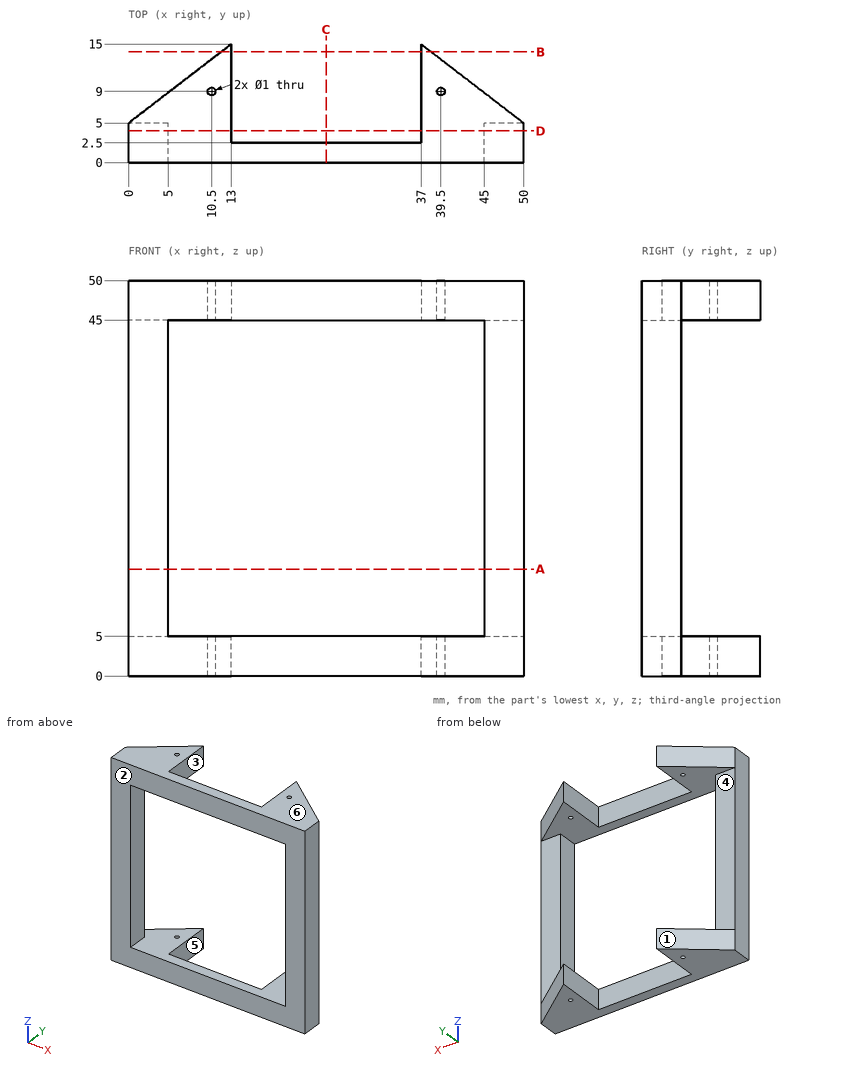
Input: dimensioned drawing with shaded views. Units: mm. Origin: part minimum x, y, z. A direction names the side the tool comes from. Give positions to 0.01 mm unless a question says otherwise; leave off trailing zeros. Order: outer loops, then holes, each group sorted by start corner. A loop starts at its lowest first (then second) coordinate and runs counter-clockwise, first axis right, second up. Notation, with made-up numbers: (79, 37) -> (114, 37) arc R19 cw to (114, 69) -> close; hole circle Ø10 at (20, -21). An arc over 180 degrees is marked (long way). Answer as a JSON object with one key per item and string values.
Q1. Access query for the marked faces 4, 5 and 6. Directions: +Z, -Z, +X, -X, +Y, -Y. A direction counts if a zero-diameter tool reaches every point of the face in a straight line with its end or side. Return the directions, or none.
Entries:
{"face 4": "+X, -X, +Y", "face 5": "+Z, -Z, +Y", "face 6": "+Z, +X, -X, +Y, -Y"}
Q2. Draft query along X for the marked faces 1, 2 and 3. Return one class per face: released by +X, released by -X, zero draft, split by the parting line, or undercut.
Entries:
{"face 1": "released by -X", "face 2": "zero draft", "face 3": "undercut"}
Q3. Section B-B (y = 14). Output: boundary loops of the cut face in (x, z), plus the area to 3 significant figures.
Entries:
{"outline": "(11.7, 0) -> (13, 0) -> (13, 5) -> (11.7, 5) -> close; (11.7, 45) -> (13, 45) -> (13, 50) -> (11.7, 50) -> close; (37, 0) -> (38.3, 0) -> (38.3, 5) -> (37, 5) -> close; (37, 45) -> (38.3, 45) -> (38.3, 50) -> (37, 50) -> close", "area": "26.0 mm^2"}
Q4. Section A-A (z = 13.5). Output: boundary loops of the cut face in (x, y).
Entries:
{"outline": "(0, 0) -> (5, 0) -> (5, 5) -> (0, 5) -> close; (45, 0) -> (50, 0) -> (50, 5) -> (45, 5) -> close"}
Q5. Section D-D (y = 4). Output: boundary loops of the cut face in (x, z), plus the area to 3 significant figures.
Entries:
{"outline": "(0, 0) -> (13, 0) -> (13, 5) -> (5, 5) -> (5, 45) -> (13, 45) -> (13, 50) -> (0, 50) -> close; (37, 0) -> (50, 0) -> (50, 50) -> (37, 50) -> (37, 45) -> (45, 45) -> (45, 5) -> (37, 5) -> close", "area": "660 mm^2"}
Q6. First-contact query: pin 1 (2.5 mm diameter, centred on y = 6.5, z = 3.5, fed in from +X) (3 decimals); pin 2 (4 mm diameter, centred on y = 7.5, z = 47.5, fed in from +X); pin 3 (1.5 mm diameter, centred on x = 28.5, z = 47, fed in from +Y). Flat tips, straight axial feed; report the tip coordinate or a pass-through.
Entries:
{"pin 1": "stops at x = 49.675", "pin 2": "stops at x = 49.35", "pin 3": "stops at y = 2.5"}
Q7. Material intervals for probe 1 along Z at (x, y) = (9.5, 7.75); probe 2 along X at (y, z) = (14, 3), sorted ascending.
Entries:
{"probe 1": "z = 0 to 5, 45 to 50", "probe 2": "x = 11.7 to 13, 37 to 38.3"}
Q8. Section C-C (x = 25). Output: boundary loops of the cut face in (y, z).
Entries:
{"outline": "(0, 0) -> (2.5, 0) -> (2.5, 5) -> (0, 5) -> close; (0, 45) -> (2.5, 45) -> (2.5, 50) -> (0, 50) -> close"}
